Work out the finished part from the listing and answer in its coordinate system (mm). Coordinates: 2 decimals unless noted, no trailing zeros. Write each loop counter-clockwise with the first axis right and the second up, starting at its lowest first coordinate (ties: lowest second). Pieces come first, ordered by that corner, then holes. Notation, with made-up numbers: (-10.75, 47) - (8.25, 47) arc R20 ccw to (8.25, 51) - close; hole circle Ø9 at (76, 80). An arc over 180 degrees is marked (long way). Use one line per item in the form item = value. Start each with the question number.
Item 1: A cutting plane is placed at B-B (y = 1.7). Give the number of separate pieces and of enclosed holes in the cut face, then the cut area to 3 significant figures.
Item 2: A cutting plane is placed at A-A (x = 31). Write down the section's boundary in (y, z).
Item 3: A cutting plane is placed at C-C (x = 85). Write down the section's boundary in (y, z), then the cut area to 3 significant figures.
Item 4: Consider probe 1 along Z at (x, y) = (37, 2.1); probe 2 along X at (y, z) = (1.45, 18.5); probe 3 along X at (y, z) = (1, 28). Determine where each line is inside the solid, lowest interval first.
Item 5: Given pin 1 (1.5 mm diameter, centred on x = 28.5, y = 1.5, fed in from +Z); pin 2 (1.5 mm diameter, centred on x = 32.5, y = 2, fed in from -Z); pin 3 (0.9 mm diameter, centred on x = 175.5, y = 1, fed in from +Z), each flat-ended and moving along its own axis, determine where each tip first touches the part or whether it passes through.
from build123d import *

# Parameters (mm, degrees)
BOSS_EXTRUDE1_DEPTH                        = 3
FILLET1_R                                  = 1
SKETCH2_R                                  = 1.6
MOTOR_DRIVER_HOLES_DEPTH                   = 204.240768548
SKETCH3_W                                  = 20
SKETCH3_H                                  = 15
MOTOR_DRIVER_ROUTING_POCKET_DEPTH          = 204.240768548
MOTOR_DRIVER_ROUTING_POCKET_FILLETS_R      = 1
MOTOR_DRIVER_ROUTING_POCKET_FILLETS_OF_M_R = 1


with BuildPart() as part:
    # Sketch1 → Boss-Extrude1 (new body)
    with BuildSketch(Plane(origin=(0, 0, 0), x_dir=(1, 0, 0), z_dir=(0, 1, 0))):
        Polygon((0, 52), (0, -52), (87.617056359, -52), (106.15, -84.1), (143.85, -84.1), (165.096489906, -47.3), (185, -47.3), (185, 47.3), (165.096489906, 47.3), (143.85, 84.1), (106.15, 84.1), (87.617056359, 52), align=None)
    extrude(amount=BOSS_EXTRUDE1_DEPTH)

    # Fillet1
    fillet1_edges = [part.edges().sort_by_distance(p)[0] for p in [
        (185, 1.5, -47.3),
        (185, 1.5, 47.3),
        (0, 1.5, 52),
        (0, 1.5, -52),
    ]]
    fillet(fillet1_edges, radius=FILLET1_R)

    # Sketch2 → Motor Driver Holes (cut, through all)
    with BuildSketch(Plane(origin=(0, 3, 0), x_dir=(1, 0, 0), z_dir=(0, 1, 0))):
        with Locations(Location((4, 18.5, 0), (0, 0, 270))):
            Circle(SKETCH2_R)
        with Locations(Location((41, 18.5, 0), (0, 0, 270))):
            Circle(SKETCH2_R)
        with Locations(Location((4, -18.5, 0), (0, 0, 270))):
            Circle(SKETCH2_R)
        with Locations(Location((41, -18.5, 0), (0, 0, 270))):
            Circle(SKETCH2_R)
    extrude(amount=-MOTOR_DRIVER_HOLES_DEPTH, mode=Mode.SUBTRACT)

    # Sketch3 → Motor Driver Routing Pocket (cut, through all)
    with BuildSketch(Plane(origin=(0, 3, 0), x_dir=(1, 0, 0), z_dir=(0, 1, 0))):
        with Locations((28, 32.5)):
            Rectangle(SKETCH3_W, SKETCH3_H)
    motor_driver_routing_pocket = extrude(amount=-MOTOR_DRIVER_ROUTING_POCKET_DEPTH, mode=Mode.SUBTRACT)

    # Motor Driver Routing Pocket Fillets
    motor_driver_routing_pocket_fillets_edges = [part.edges().sort_by_distance(p)[0] for p in [
        (38, 1.5, -40),
        (38, 1.5, -25),
        (18, 1.5, -25),
        (18, 1.5, -40),
    ]]
    fillet(motor_driver_routing_pocket_fillets_edges, radius=MOTOR_DRIVER_ROUTING_POCKET_FILLETS_R)

    # Mirror1: Motor Driver Routing Pocket across plane
    add(motor_driver_routing_pocket.mirror(Plane.XY), mode=Mode.SUBTRACT)

    # Motor Driver Routing Pocket Fillets of M
    motor_driver_routing_pocket_fillets_of_m_edges = [part.edges().sort_by_distance(p)[0] for p in [
        (38, 1.5, 40),
        (38, 1.5, 25),
        (18, 1.5, 25),
        (18, 1.5, 40),
    ]]
    fillet(motor_driver_routing_pocket_fillets_of_m_edges, radius=MOTOR_DRIVER_ROUTING_POCKET_FILLETS_OF_M_R)


solid = part.part
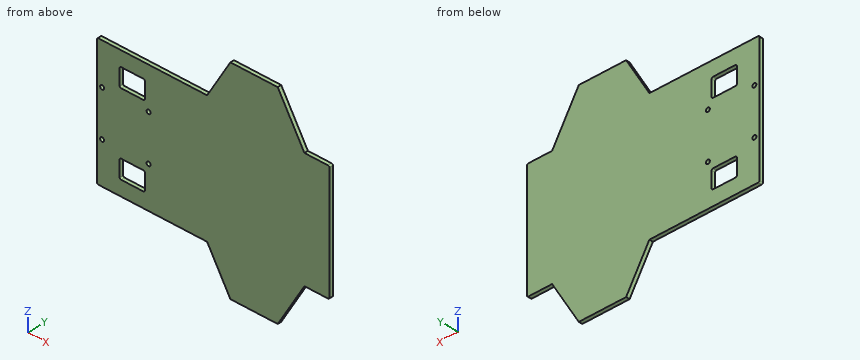
Answer:
q1.separate_pieces = 1
q1.enclosed_holes = 6
q1.area = 22,000 mm²
q2.outline = (0, -52) - (3, -52) - (3, -40) - (0, -40) - close; (0, -25) - (3, -25) - (3, 25) - (0, 25) - close; (0, 40) - (3, 40) - (3, 52) - (0, 52) - close
q3.outline = (0, -52) - (3, -52) - (3, 52) - (0, 52) - close
q3.area = 312 mm²
q4.probe_1 = -52 to -40, -25 to 25, 40 to 52
q4.probe_2 = 0 to 2.4, 5.6 to 39.4, 42.6 to 185
q4.probe_3 = 0 to 18, 38 to 185
q5.pin_1 = 52
q5.pin_2 = -52
q5.pin_3 = 47.3
